Build history of the part. All positions in model axes, mm. Face numbers are marked on the shaded views. Round coordinates to 2 decimals unless told otherwise and drop trailing zeros. Write each loop counter-clockwise with the first axis right and the second up, starting at its lowest first coordinate (ties: lowest second). Pieces come first, ordered by that corner, then holes. Notation, with made-up numbers: (-15.5, -20) -> (5.5, -20) arc R24 ccw to (5.5, 3) -> close; hole circle Ø2 at (-6.75, -25). An arc over 180 degrees is marked (long way). Return JSON: item names as keys, results as strings.
from build123d import *

# Parameters (mm, degrees)
SKETCH2_R           = 3.475
BOSS_EXTRUDE2_DEPTH = 14.575
SKETCH3_R           = 1.475
CUT_EXTRUDE1_DEPTH  = 10
CUT_EXTRUDE2_START  = -10
SKETCH4_R           = 1.475
CUT_EXTRUDE2_DEPTH  = 10
BOSS_EXTRUDE3_DEPTH = 14.575
SKETCH6_W           = 6.95
SKETCH6_H           = 14.575
BOSS_EXTRUDE4_DEPTH = 0.2


with BuildPart() as part:
    # Sketch2 → Boss-Extrude2 (new body)
    with BuildSketch(Plane.XY):
        Circle(SKETCH2_R)
    extrude(amount=BOSS_EXTRUDE2_DEPTH)

    # Sketch3 → Cut-Extrude1 (cut)
    with BuildSketch(Plane.XY.offset(14.575)):
        Circle(SKETCH3_R)
    extrude(amount=-CUT_EXTRUDE1_DEPTH, mode=Mode.SUBTRACT)

    # Sketch4 → Cut-Extrude2 (cut)
    with BuildSketch(Plane(origin=(0, 0, 0), x_dir=(-1, 0, 0), z_dir=(0, 0, -1)).offset(CUT_EXTRUDE2_START)):
        with Locations(Location((0, 0, 0), (0, 0, 180))):
            Circle(SKETCH4_R)
    extrude(amount=CUT_EXTRUDE2_DEPTH, mode=Mode.SUBTRACT)

    # Sketch5 → Boss-Extrude3 (add)
    with BuildSketch(Plane(origin=(0, 0, 0), x_dir=(-1, 0, 0), z_dir=(0, 0, -1))):
        with BuildLine():
            ThreePointArc((0, -3.475), (-2.457196065, -2.457196065), (-3.475, 0))
            Line((-3.475, 0), (-3.475, -3.475))
            Line((-3.475, -3.475), (0, -3.475))
        make_face()
        with BuildLine():
            Line((3.475, -3.475), (3.475, 0))
            ThreePointArc((3.475, 0), (2.457196065, -2.457196065), (0, -3.475))
            Line((0, -3.475), (3.475, -3.475))
        make_face()
    extrude(amount=-BOSS_EXTRUDE3_DEPTH)

    # Sketch6 → Boss-Extrude4 (add)
    with BuildSketch(Plane.XZ.offset(3.475)):
        with Locations((0, 7.2875)):
            Rectangle(SKETCH6_W, SKETCH6_H)
    extrude(amount=BOSS_EXTRUDE4_DEPTH)


solid = part.part
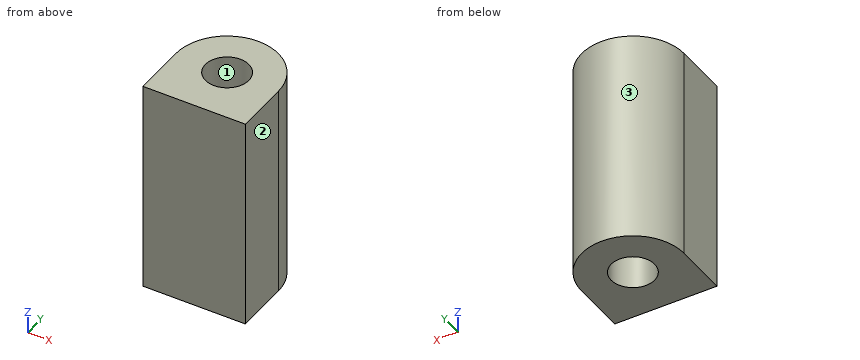
Q1. Saw through at A-A on x = 0. List the corners of the cut face in (y, z) (3 decimals).
Verdict:
{"outline": "(-3.675, 0) -> (-1.475, 0) -> (-1.475, 14.575) -> (-3.675, 14.575) -> close; (1.475, 0) -> (3.475, 0) -> (3.475, 14.575) -> (1.475, 14.575) -> close"}
Q2. Saw through at D-D on x = -2.25. List the corners of the cut face in (y, z) (3 decimals).
Verdict:
{"outline": "(-3.675, 0) -> (2.648, 0) -> (2.648, 14.575) -> (-3.675, 14.575) -> close"}
Q3. Wall check: L1, parallel to Y at x = 0, z = 3.5 (3 decimals); L2, parallel to X at y = 0, z = 5 (3 decimals); L3, parallel to Y at x = -1, z = 4.75 (3 decimals). Give the ranges that are in metal, low to high.
Verdict:
{"L1": "y = -3.675 to -1.475, 1.475 to 3.475", "L2": "x = -3.475 to -1.475, 1.475 to 3.475", "L3": "y = -3.675 to -1.084, 1.084 to 3.328"}
Q4. Saw through at B-B on y = -0.25. List the corners of the cut face in (x, z) (3 decimals), then the cut area to 3 significant figures.
Verdict:
{"outline": "(-3.475, 0) -> (-1.454, 0) -> (-1.454, 14.575) -> (-3.475, 14.575) -> close; (1.454, 0) -> (3.475, 0) -> (3.475, 14.575) -> (1.454, 14.575) -> close", "area": "58.9 mm²"}
Q5. Saw through at C-C on z = 13.75. List the corners of the cut face in (x, y) (3 decimals).
Verdict:
{"outline": "(-3.475, -3.675) -> (3.475, -3.675) -> (3.475, 0) arc R3.475 ccw to (-3.475, 0) -> close; hole circle Ø2.95 at (0, 0)"}
Q6. Two-plate mould, pull along X, no slides. Class the marked faces 1, 2 and 3: +X half, -X half, draft (parallel to the pull), parting line (faces both ways), or undercut.
Verdict:
{"face 1": "undercut", "face 2": "+X half", "face 3": "parting line"}
Q7. Pin check, flat tips, straight feed: pin 1 Ø1 at (x, z) = (2.5, 7) entering from +Y; pin 2 Ø1 at (y, z) = (1.5, 4.5) entering from -X; pin 3 Ø4 at (x, y) = (0, 0) entering from +Z (3 decimals); pin 4 Ø1 at (x, z) = (1, 10) entering from +Y. Stop position of each tip, or through.
Verdict:
{"pin 1": "stops at y = 2.84", "pin 2": "stops at x = -3.33", "pin 3": "stops at z = 14.575", "pin 4": "stops at y = 3.44"}
